from build123d import *

# Parameters (mm, degrees)
SKETCH1_W           = 16.51
SKETCH1_H           = 10.16
SKETCH1_W_2         = 31.75
BOSS_EXTRUDE1_DEPTH = 5.08
SKETCH2_W           = 5.08
SKETCH2_H           = 20.32
BOSS_EXTRUDE2_DEPTH = 33.02
SKETCH4_R           = 2.54
SKETCH4_R_2         = 1.0795
BOSS_EXTRUDE3_DEPTH = 5.08
SKETCH5_R           = 1.0795
CUT_EXTRUDE1_DEPTH  = 39.1
SKETCH6_R           = 1.0795
CUT_EXTRUDE2_DEPTH  = 8.89


with BuildPart() as part:
    # Sketch1 → Boss-Extrude1 (new body)
    with BuildSketch(Plane(origin=(0, 0, 0), x_dir=(1, 0, 0), z_dir=(0, 1, 0))):
        Polygon((-42.545, 28.956), (-37.465, 28.956), (-37.465, 10.16), (37.465, 10.16), (37.465, 28.956), (42.545, 28.956), (42.545, -28.956), (37.465, -28.956), (37.465, -10.16), (-37.465, -10.16), (-37.465, -28.956), (-42.545, -28.956), align=None)
        with Locations((29.21, 0)):
            Rectangle(SKETCH1_W, SKETCH1_H, mode=Mode.SUBTRACT)
        with Locations((-29.21, 0)):
            Rectangle(SKETCH1_W, SKETCH1_H, mode=Mode.SUBTRACT)
        Rectangle(SKETCH1_W_2, SKETCH1_H, mode=Mode.SUBTRACT)
    extrude(amount=BOSS_EXTRUDE1_DEPTH)

    # Sketch2 → Boss-Extrude2 (add)
    with BuildSketch(Plane.XZ):
        with Locations((-18.415, 0)):
            Rectangle(SKETCH2_W, SKETCH2_H)
        with Locations((18.415, 0)):
            Rectangle(SKETCH2_W, SKETCH2_H)
    extrude(amount=BOSS_EXTRUDE2_DEPTH)

    # Sketch4 → Boss-Extrude3 (add)
    with BuildSketch(Plane(origin=(0, 5.08, 0), x_dir=(1, 0, 0), z_dir=(0, 1, 0))):
        with Locations((-40.005, 26.416)):
            Circle(SKETCH4_R)
        with Locations((-40.005, 26.416)):
            Circle(SKETCH4_R_2, mode=Mode.SUBTRACT)
        with Locations((-40.005, -26.416)):
            Circle(SKETCH4_R)
        with Locations((-40.005, -26.416)):
            Circle(SKETCH4_R_2, mode=Mode.SUBTRACT)
        with Locations((40.005, -26.416)):
            Circle(SKETCH4_R)
        with Locations((40.005, -26.416)):
            Circle(SKETCH4_R_2, mode=Mode.SUBTRACT)
        with Locations((40.005, 26.416)):
            Circle(SKETCH4_R)
        with Locations((40.005, 26.416)):
            Circle(SKETCH4_R_2, mode=Mode.SUBTRACT)
    extrude(amount=BOSS_EXTRUDE3_DEPTH)

    # Sketch5 → Cut-Extrude1 (cut, through all)
    with BuildSketch(Plane(origin=(0, 5.08, 0), x_dir=(1, 0, 0), z_dir=(0, 1, 0))):
        with Locations((-40.005, -26.416)):
            Circle(SKETCH5_R)
        with Locations((-40.005, 26.416)):
            Circle(SKETCH5_R)
        with Locations((40.005, 26.416)):
            Circle(SKETCH5_R)
        with Locations((40.005, -26.416)):
            Circle(SKETCH5_R)
    extrude(amount=-CUT_EXTRUDE1_DEPTH, mode=Mode.SUBTRACT)

    # Sketch6 → Cut-Extrude2 (cut)
    with BuildSketch(Plane.XZ.offset(33.02)):
        with Locations((-18.415, 7.62)):
            Circle(SKETCH6_R)
        with Locations((-18.415, -7.62)):
            Circle(SKETCH6_R)
        with Locations((18.415, 7.62)):
            Circle(SKETCH6_R)
        with Locations((18.415, -7.62)):
            Circle(SKETCH6_R)
    extrude(amount=-CUT_EXTRUDE2_DEPTH, mode=Mode.SUBTRACT)


solid = part.part
Build history of the part. All positions in model axes, mm. A direction names the side the tool comes from. Coordinates: 2 decimals unless noted, no trailing zeros. Order: outer loops, then holes, each group sorted by start corner. A loop starts at its lowest first (then second) coordinate and runs counter-clockwise, first axis right, second up. Notation, with made-up numbers: (37, -17.75) - (59, -17.75) arc R6 cw to (59, -10.75) - close; hole circle Ø8 at (-13, -0.5). An arc over 180 degrees is marked (long way). Write item = value, one per line. Start each with the question number.
1) Saw through at B-B on z = 20. Write the cut outline in (x, y) (3 decimals), then the cut area to 3 significant figures.
2) 3-axis set-ups, long thin cutter, end or side, ignore diameter. For faces 4 (the face through (-37.582, 7.584, 25.653)), 5 (the face through (42, 5.08, 28.3)), 6 (the face through (37.465, 3, 20)), 7 (the face through (-39, 0, 0)), 8 (the face through (29, 3, -5.08)): which of +Z, -Z, +X, -X, +Y, -Y reach the whole face in a straight line?
3) Saw through at C-C on y = 6. Write the cut outline in (x, z) (1 decimal), then the cut area to 3 significant figures.
4) Saw through at D-D on z = -2.5. Write the cut outline in (x, y) (3 decimals).
5) Wall check: line 1 along X through (y, z) = (-30.5, 7.5) (3 decimals); line 2 along X through (y, z) = (-24, 9) (3 decimals); line 3 along Z through (x, y) = (10.5, 4). Give the ranges that are in metal, low to high. Write a range as from..to.
6) Two-plate mould, pull along Z, no slides. Class faces 1 (the face through (17.62, -28.64, 8.35)), 2 (the face through (40, 3, -28.956)), 3 (the face through (42, 5.08, -28.4)): pulls with the +Z half, pulls with the -Z half, needs draft (parallel to the pull), parting line crosses it, or undercut.
7) Flat gauge pins, fed straight in: pin 1 Ø22.5 at (y, z) = (-14, -4) entering from +X (3 decimals); pin 2 Ø19 at (x, y) = (16.5, -9) entering from +Z; pin 3 Ø1.5 at (x, y) = (30, 1.5) entering from -Z; pin 4 Ø1.9 at (x, z) = (40.005, 26.416) entering from -Y. Where does each tip first touch, or does it go through?
8) Saw through at A-A on y = -19.5. Write the cut outline in (x, z) (3 decimals), then the cut area to 3 significant figures.
From the geometry:
q1.outline = (-42.545, 0) - (-37.465, 0) - (-37.465, 5.08) - (-42.545, 5.08) - close; (37.465, 0) - (42.545, 0) - (42.545, 5.08) - (37.465, 5.08) - close
q1.area = 51.6 mm^2
q2.face_4 = +Y
q2.face_5 = +Z, +X, +Y
q2.face_6 = +Z, +Y, -Y
q2.face_7 = +Z, -Z, -X, -Y
q2.face_8 = +Y, -Y
q3.outline = circle Ø5.1 at (-40, -26.4); circle Ø5.1 at (-40, 26.4); circle Ø5.1 at (40, -26.4); circle Ø5.1 at (40, 26.4); hole circle Ø2.2 at (-40, -26.4); hole circle Ø2.2 at (-40, 26.4); hole circle Ø2.2 at (40, -26.4); hole circle Ø2.2 at (40, 26.4)
q3.area = 66.4 mm^2
q4.outline = (-42.545, 0) - (-37.465, 0) - (-37.465, 5.08) - (-42.545, 5.08) - close; (-20.955, -33.02) - (-15.875, -33.02) - (-15.875, 5.08) - (-20.955, 5.08) - close; (15.875, -33.02) - (20.955, -33.02) - (20.955, 5.08) - (15.875, 5.08) - close; (37.465, 0) - (42.545, 0) - (42.545, 5.08) - (37.465, 5.08) - close
q5.line_1 = -20.955..-19.488, -17.342..-15.875, 15.875..17.342, 19.488..20.955
q5.line_2 = -20.955..-15.875, 15.875..20.955
q5.line_3 = -10.16..-5.08, 5.08..10.16
q6.face_1 = undercut
q6.face_2 = pulls with the -Z half
q6.face_3 = needs draft
q7.pin_1 = 20.955
q7.pin_2 = 10.16
q7.pin_3 = -10.16
q7.pin_4 = through
q8.outline = (-20.955, -10.16) - (-15.875, -10.16) - (-15.875, 10.16) - (-20.955, 10.16) - close; (15.875, -10.16) - (20.955, -10.16) - (20.955, 10.16) - (15.875, 10.16) - close
q8.area = 206 mm^2
